from build123d import *

# Parameters (mm, degrees)
F3_SIZE  = 0.5
F2_R     = 2.5
F4_DEPTH = 6
F5_COUNT = 8
F8_DEPTH = 4


with BuildPart() as f1:
    # F0 (on Front) → F1 (revolve)
    with BuildSketch(Plane.XZ):
        Polygon((1.5, 6), (1.5, 0), (9, 0), (9, 4), (6, 4), (4, 6), align=None)
    revolve(axis=Axis((0, 0, 3.871229), (0, 0, -1)))

    # F3
    f3_edges = [f1.edges().sort_by_distance(p)[0] for p in [
        (-9, 0, 4),
        (-9, 0, 0),
    ]]
    chamfer(f3_edges, length=F3_SIZE)


with BuildPart() as f4:
    # F2 (on Top) → F4 (new body, through all)
    with BuildSketch(Plane.XY):
        with Locations((0, 10)):
            Circle(F2_R)
    extrude(amount=F4_DEPTH)


with BuildPart() as f5_1:
    # F5: instance of F4
    add(f4.part.rotate(Axis((0, 0, 6), (0, 0, -1)), 1 * 360 / F5_COUNT))


with BuildPart() as f5_2:
    # F5: instance of F4
    add(f4.part.rotate(Axis((0, 0, 6), (0, 0, -1)), 2 * 360 / F5_COUNT))


with BuildPart() as f5_3:
    # F5: instance of F4
    add(f4.part.rotate(Axis((0, 0, 6), (0, 0, -1)), 3 * 360 / F5_COUNT))


with BuildPart() as f5_4:
    # F5: instance of F4
    add(f4.part.rotate(Axis((0, 0, 6), (0, 0, -1)), 4 * 360 / F5_COUNT))


with BuildPart() as f5_5:
    # F5: instance of F4
    add(f4.part.rotate(Axis((0, 0, 6), (0, 0, -1)), 5 * 360 / F5_COUNT))


with BuildPart() as f5_6:
    # F5: instance of F4
    add(f4.part.rotate(Axis((0, 0, 6), (0, 0, -1)), 6 * 360 / F5_COUNT))


with BuildPart() as f5_7:
    # F5: instance of F4
    add(f4.part.rotate(Axis((0, 0, 6), (0, 0, -1)), 7 * 360 / F5_COUNT))


with BuildPart() as f1_1:
    add(f1.part)

    # F6: cut F4, F5_1, F5_2, F5_3, F5_4, F5_5, F5_6, F5_7
    add(f4.part, mode=Mode.SUBTRACT)
    add(f5_1.part, mode=Mode.SUBTRACT)
    add(f5_2.part, mode=Mode.SUBTRACT)
    add(f5_3.part, mode=Mode.SUBTRACT)
    add(f5_4.part, mode=Mode.SUBTRACT)
    add(f5_5.part, mode=Mode.SUBTRACT)
    add(f5_6.part, mode=Mode.SUBTRACT)
    add(f5_7.part, mode=Mode.SUBTRACT)

    # F7 (on face) → F8 (cut)
    with BuildSketch(Plane(origin=(0, 0, 0), x_dir=(1, 0, 0), z_dir=(0, 0, -1))):
        Polygon((-1.587713, 2.75), (-3.175426, 0), (-1.587713, -2.75), (1.587713, -2.75), (3.175426, 0), (1.587713, 2.75), align=None)
    extrude(amount=-F8_DEPTH, mode=Mode.SUBTRACT)


solid = f1_1.part
Here's how the part is built. I have some questions about the finished solid (model axes, mm). A direction names the side the tool comes from. Coordinates: 2 decimals unless noted, no trailing zeros. Loops run counter-clockwise (first coordinate to the right, second up) from the corner with the lowest first, then second, coordinate; pieces in that order, holes last.
1. Imagine slicing it at B-B, the plane z = 1. Please give me the cut outline in (x, y).
2. Imagine slicing it at C-C, the plane z = 4.75. Please give me the cut outline in (x, y).
3. Imagine slicing it at A-A, the plane x = 0. Please give me the cut outline in (y, z).
4. For P1, Ø10, axis at x = 6, y = -1, coming from the +Z side; P2, Ø1.6, axis at x = -0.5, z = 2, coming from the -Y side; P3, Ø3, axis at y = -4.5, z = 1, coming from the +X side; P4, Ø2.5, axis at x = 0, y = 0, coming from the +Z side, each with a flat end and sliding along its axis, tell me the tip position at first contact or that it passes through.
5. If we mould it in two halves opening along Y, with no side actions, what happens to faces 1 (the cylindrical face through (3.46, -8.31, 2.02)), 2 (the cylindrical face through (-7.5, 0, 2)), 3 (the cylindrical face through (-8.32, 3.43, 2.02))? For each: pulls with the +Y half, pulls with the -Y half, needs draft (parallel to the pull), parting line crosses it, or undercut.
6. Imagine slicing it at D-D, the plane x = -6.25. Please give me the cut outline in (y, z), and give its area (3 significant figures).
7. I need wall thicknesses on L1, parallel to Z at x = -1.5, y = -2.5; L2, parallel to X at y = -1, z = 4.75; L3, parallel to X at y = 0, z = 4.6. Which ranges of each line are inside material? Lowest first, please.
8. For faces 4 (the cylindrical face through (3.43, 8.32, 2.02)), 5 (the flat face through (0, -2.75, 2)), which set-ups out of +Z, -Z, +X, -X, +Y, -Y let a thin tool reach every point of the face, with its end or its side?
Taken from the geometry:
1. outline: (-8.74, -2.16) arc R9 ccw to (-7.7, -4.65) arc R2.5 cw to (-4.65, -7.7) arc R9 ccw to (-2.16, -8.74) arc R2.5 cw to (2.16, -8.74) arc R9 ccw to (4.65, -7.7) arc R2.5 cw to (7.7, -4.65) arc R9 ccw to (8.74, -2.16) arc R2.5 cw to (8.74, 2.16) arc R9 ccw to (7.7, 4.65) arc R2.5 cw to (4.65, 7.7) arc R9 ccw to (2.16, 8.74) arc R2.5 cw to (-2.16, 8.74) arc R9 ccw to (-4.65, 7.7) arc R2.5 cw to (-7.7, 4.65) arc R9 ccw to (-8.74, 2.16) arc R2.5 cw to start; hole (-3.18, 0) - (-1.59, -2.75) - (1.59, -2.75) - (3.18, 0) - (1.59, 2.75) - (-1.59, 2.75) - close
2. outline: circle Ø10.5 at (0, 0); hole circle Ø3 at (0, 0)
3. outline: (-7.5, 0) - (-2.75, 0) - (-2.75, 4) - (-1.5, 4) - (-1.5, 6) - (-4, 6) - (-6, 4) - (-7.5, 4) - close; (1.5, 4) - (2.75, 4) - (2.75, 0) - (7.5, 0) - (7.5, 4) - (6, 4) - (4, 6) - (1.5, 6) - close
4. P1: stops at z = 6
4. P2: stops at y = -7.86
4. P3: stops at x = 8.49
4. P4: passes through
5. face 1: pulls with the -Y half
5. face 2: undercut
5. face 3: pulls with the +Y half
6. outline: (-4.71, 0) - (4.71, 0) - (4.71, 4) - (-4.71, 4) - close
6. area: 37.7 mm2
7. L1: z = 4 to 6
7. L2: x = -5.15 to -1.12, 1.12 to 5.15
7. L3: x = -5.4 to -1.5, 1.5 to 5.4
8. face 4: +Z, -Z, +X, +Y
8. face 5: -Z
